Autodesk Inventor part; units mm, degrees
ref_plane "YZ Plane" through (0, 0, 0) normal (1, 0, 0) x (0, 1, 0)
ref_plane "XZ Plane" through (0, 0, 0) normal (0, 1, 0) x (-1, 0, 0)
ref_plane "XY Plane" through (0, 0, 0) normal (0, 0, 1) x (1, 0, 0)
sketch "Sketch1" plane through (0, 0, 0) normal (0, 0, 1) x (1, 0, 0)
  circle A0 centre (0, 0) radius 3.175
  dimension "d0" = 6.35
extrude "Extrusion1" add sketch "Sketch1" along normal blind 0.635
sketch "Sketch2" plane through (0, 0, 0.635) normal (0, 0, 1) x (1, 0, 0)
  circle A0 centre (0, 0) radius 3.175
  circle A1 centre (0, 0) radius 2.921
  dimension "d6" = 5.842
extrude "Extrusion2" add sketch "Sketch2" along normal blind 0.7366 contours A1
sketch "Sketch3" plane through (0, 0, 1.3716) normal (0, 0, 1) x (1, 0, 0)
  circle A0 centre (0, 0) radius 2.921
  circle A1 centre (0, 0) radius 3.175
  dimension "d10" = 6.35
extrude "Extrusion3" add sketch "Sketch3" along normal blind 37.0205 contours A0 | A1
sketch "Sketch4" plane through (0, 0, 38.3921) normal (0, 0, 1) x (1, 0, 0)
  circle A0 centre (0, 0) radius 3.175
  circle A1 centre (0, 0) radius 2.921
  dimension "d13" = 5.842
extrude "Extrusion4" add sketch "Sketch4" along normal blind 0.7366 contours A1
sketch "Sketch5" plane through (0, 0, 39.1287) normal (0, 0, 1) x (1, 0, 0)
  circle A0 centre (0, 0) radius 2.921
  circle A1 centre (0, 0) radius 3.175
  dimension "d16" = 6.35
extrude "Extrusion5" add sketch "Sketch5" along normal blind 0.635 contours A0 | A1
chamfer "Chamfer1" distance 0.127 angle 45 2 edges at (-3.175, 0, 0) (-3.175, 0, 39.7637)
properties part number "Belt Shaft"
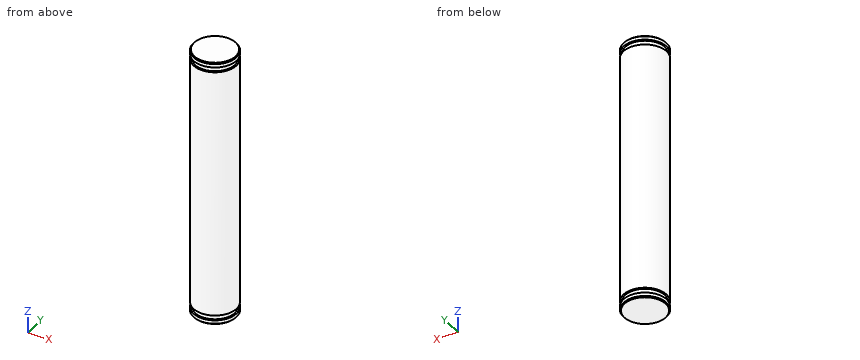
Geometry: final body of the model. Coordinates: model frame, mm. Coordinates: 2 decimals unless noted, no trailing zeros. Order: outer loops, then holes, each group sorted by start corner. A loop starts at its lowest first (then second) coordinate and runs counter-clockwise, first axis right, second up. Notation, with made-up numbers: M 28.25,80.25 L 86.25,80.25 A27 cw 86.25,118.25 Z; hole C 39,83.5 d2. An arc over 180 degrees is marked long. Answer in a Markdown table with one row per item. Add a question column.
Q1. Contact query for flat-ended pins moving along their axis: P1, Ø2, axis at x = 1.5, z = 29.5, coming from the -Y side; P2, Ø2, axis at y = -2, z = 21.5, coming from the +X side; P3, Ø1.5, axis at x = 2, z = 4.5, coming from the +Y side. Output: stop coordinate, or through.
Q2. Line query: L1, parallel to Z at x = -3, y = -0.25 (3 decimals); L2, parallel to X at y = 2.5, z = 22.5; L3, parallel to Y at x = 0.5, z = 28. Output: solid intervals per line, ascending.
Q3. Section query A-A on z = 21.5. Return the cut outline in (x, y) (3 decimals), and give its area (3 significant figures).
Completed:
| question | item | result |
|---|---|---|
| 1 | P1 | stops at y = -3.14 |
| 1 | P2 | stops at x = 3.01 |
| 1 | P3 | stops at y = 2.92 |
| 2 | L1 | z = 0 to 0.635, 1.372 to 38.392, 39.129 to 39.764 |
| 2 | L2 | x = -1.96 to 1.96 |
| 2 | L3 | y = -3.14 to 3.14 |
| 3 | outline | C 0,0 d6.35 |
| 3 | area | 31.7 mm2 |
